Verification items for the finished model (mm, model axes). Round coordinates to 2 decimals unless told otherwise and drop trailing zeros. Write each loop counter-clockwise with the first axis right and the second up, starting at its lowest first coordinate (ties: lowest second). Pieces come first, ordered by that corner, then holes. Notation, with made-up numbers: M 62,29.25 L 103,29.25 A17 ccw 103,42.25 Z; hole C -10,-15.75 d7. An arc over 180 degrees is marked long. One line per item, written item: value. Start each with the question number.
Item 1: Section check A-A, the plane z = 1.7. Record the cut outline in (x, y) (3 decimals), then the cut area to 3 significant figures.
Item 2: Thickness scan on probe 1 along X at (y, z) = (13.5, 1.45) (3 decimals); probe 2 along X at (y, z) = (-10.5, 0.2). Record the ranges inside material, lowest first. Write a range as from..to.
Item 3: Gauge pin test, flat ends, axial feed: pin 1 (1 mm diameter, centred on y = 26.5, z = 1, fed in from +X) (3 decimals); pin 2 (1.6 mm diameter, centred on x = 26, z = 1.5, fed in from -Y) (3 decimals). Record the tip position at first contact, or that the pin passes through.
Item 4: Section check B-B, the plane x = 29. Record the cut outline in (y, z) (3 decimals).
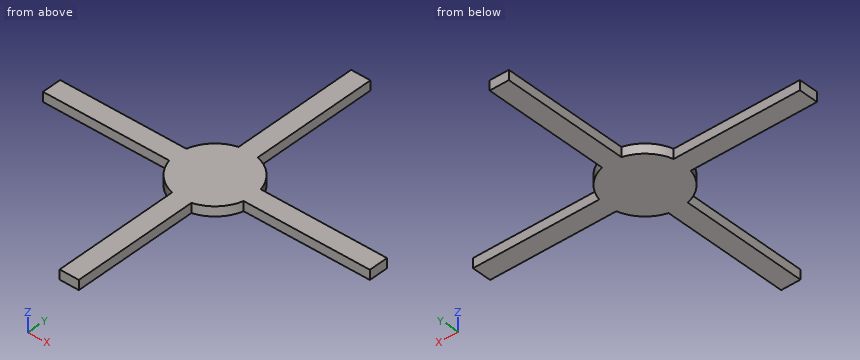
from build123d import *

# Parameters (mm, degrees)
F0_W     = 6.35
F0_H     = 6.35
F1_DEPTH = 3.175


with BuildPart() as f1:
    # F0 (on Top) → F1 (new body)
    with BuildSketch(Plane.XY):
        with BuildLine():
            Line((-12.2967221242, 3.175), (-53.975, 3.175))
            Line((-53.975, 3.175), (-53.975, -3.175))
            Line((-53.975, -3.175), (-12.2967221242, -3.175))
            ThreePointArc((-12.2967221242, -3.175), (-12.7, 0), (-12.2967221242, 3.175))
        make_face()
        with BuildLine():
            Line((53.975, 3.175), (12.2967221242, 3.175))
            ThreePointArc((12.2967221242, 3.175), (12.5987771426, 1.6002545145), (12.7, 0))
            ThreePointArc((12.7, 0), (12.5987771426, -1.6002545145), (12.2967221242, -3.175))
            Line((12.2967221242, -3.175), (53.975, -3.175))
            Line((53.975, -3.175), (53.975, 3.175))
        make_face()
        with BuildLine():
            ThreePointArc((3.175, -12.2967221242), (0, -12.7), (-3.175, -12.2967221242))
            Line((-3.175, -12.2967221242), (-3.175, -53.975))
            Line((-3.175, -53.975), (3.175, -53.975))
            Line((3.175, -53.975), (3.175, -12.2967221242))
        make_face()
        with BuildLine():
            Line((-3.175, 53.975), (-3.175, 12.2967221242))
            ThreePointArc((-3.175, 12.2967221242), (0, 12.7), (3.175, 12.2967221242))
            Line((3.175, 12.2967221242), (3.175, 53.975))
            Line((3.175, 53.975), (-3.175, 53.975))
        make_face()
        with BuildLine():
            ThreePointArc((-3.175, 12.2967221242), (-8.9802561211, 8.9802561211), (-12.2967221242, 3.175))
            Line((-12.2967221242, 3.175), (-3.175, 3.175))
            Line((-3.175, 3.175), (-3.175, 12.2967221242))
        make_face()
        with BuildLine():
            Line((3.175, 12.2967221242), (3.175, 3.175))
            Line((3.175, 3.175), (12.2967221242, 3.175))
            ThreePointArc((12.2967221242, 3.175), (8.9802561211, 8.9802561211), (3.175, 12.2967221242))
        make_face()
        with BuildLine():
            Line((-3.175, -3.175), (-12.2967221242, -3.175))
            ThreePointArc((-12.2967221242, -3.175), (-8.9802561211, -8.9802561211), (-3.175, -12.2967221242))
            Line((-3.175, -12.2967221242), (-3.175, -3.175))
        make_face()
        with BuildLine():
            Line((12.2967221242, -3.175), (3.175, -3.175))
            Line((3.175, -3.175), (3.175, -12.2967221242))
            ThreePointArc((3.175, -12.2967221242), (8.9802561211, -8.9802561211), (12.2967221242, -3.175))
        make_face()
        with BuildLine():
            Line((-3.175, 3.175), (-12.2967221242, 3.175))
            ThreePointArc((-12.2967221242, 3.175), (-12.7, 0), (-12.2967221242, -3.175))
            Line((-12.2967221242, -3.175), (-3.175, -3.175))
            Line((-3.175, -3.175), (-3.175, 3.175))
        make_face()
        with BuildLine():
            Line((-3.175, 12.2967221242), (-3.175, 3.175))
            Line((-3.175, 3.175), (3.175, 3.175))
            Line((3.175, 3.175), (3.175, 12.2967221242))
            ThreePointArc((3.175, 12.2967221242), (0, 12.7), (-3.175, 12.2967221242))
        make_face()
        with BuildLine():
            Line((12.2967221242, 3.175), (3.175, 3.175))
            Line((3.175, 3.175), (3.175, -3.175))
            Line((3.175, -3.175), (12.2967221242, -3.175))
            ThreePointArc((12.2967221242, -3.175), (12.5987771426, -1.6002545145), (12.7, 0))
            ThreePointArc((12.7, 0), (12.5987771426, 1.6002545145), (12.2967221242, 3.175))
        make_face()
        with BuildLine():
            Line((3.175, -3.175), (-3.175, -3.175))
            Line((-3.175, -3.175), (-3.175, -12.2967221242))
            ThreePointArc((-3.175, -12.2967221242), (0, -12.7), (3.175, -12.2967221242))
            Line((3.175, -12.2967221242), (3.175, -3.175))
        make_face()
        Rectangle(F0_W, F0_H)
    extrude(amount=F1_DEPTH)


solid = f1.part
Response values:
1. outline: M -53.975,-3.175 L -12.297,-3.175 A12.7 ccw -3.175,-12.297 L -3.175,-53.975 L 3.175,-53.975 L 3.175,-12.297 A12.7 ccw 12.297,-3.175 L 53.975,-3.175 L 53.975,3.175 L 12.297,3.175 A12.7 ccw 3.175,12.297 L 3.175,53.975 L -3.175,53.975 L -3.175,12.297 A12.7 ccw -12.297,3.175 L -53.975,3.175 Z
1. area: 1,560 mm2
2. probe 1: x = -3.175..3.175
2. probe 2: x = -7.14..7.14
3. pin 1: stops at x = 3.175
3. pin 2: stops at y = -3.175
4. outline: M -3.175,0 L 3.175,0 L 3.175,3.175 L -3.175,3.175 Z
